Verification items for the finished model (mm, model axes). A direction names the side the tool comes from. Round coordinates to 2 decimals unless told otherwise and drop trailing zeros. Order: outer loops, then holes, each group sorted by start corner. A loop starts at its lowest first (then second) coordinate and runs counter-clockwise, first axis right, second up. Notation, with made-up numbers: (81.5, 10.5) -> (85.5, 10.5) arc R14 ccw to (85.5, 15.5) -> close; hole circle Ø9 at (1.25, -24). An arc over 180 degrees is marked (long way). Put each result on its own line as item: value.
```python
from build123d import *

# Parameters (mm, degrees)
SKETCH1_R           = 2.4765
BOSS_EXTRUDE1_DEPTH = 9.525
SKETCH2_R           = 3.9624
BOSS_EXTRUDE2_DEPTH = 2.38125
CUT_EXTRUDE1_DEPTH  = 2.286
FILLET1_R           = 1.5875


with BuildPart() as part:
    # Sketch1 → Boss-Extrude1 (new body)
    with BuildSketch(Plane(origin=(0, 0, 0), x_dir=(1, 0, 0), z_dir=(0, 1, 0))):
        with Locations(Location((0, 0, 0), (0, 0, 90))):
            Circle(SKETCH1_R)
    extrude(amount=BOSS_EXTRUDE1_DEPTH)

    # Sketch2 → Boss-Extrude2 (add)
    with BuildSketch(Plane.XZ):
        with Locations(Location((0, 0, 0), (0, 0, 90))):
            Circle(SKETCH2_R)
    extrude(amount=BOSS_EXTRUDE2_DEPTH)

    # Sketch3 → Cut-Extrude1 (cut)
    with BuildSketch(Plane.XZ.offset(2.38125)):
        Polygon((2.062222993, 0), (1.031111496, 1.7859375), (-1.031111496, 1.7859375), (-2.062222993, 0), (-1.031111496, -1.7859375), (1.031111496, -1.7859375), align=None)
    extrude(amount=-CUT_EXTRUDE1_DEPTH, mode=Mode.SUBTRACT)

    # Fillet1
    fillet1_edges = [part.edges().sort_by_distance(p)[0] for p in [
        (0, -2.38125, -3.9624),
    ]]
    fillet(fillet1_edges, radius=FILLET1_R)


solid = part.part
```
Item 1: Depth check by flat-ended pin: pin 1 Ø1.5 at (y, z) = (3, 2.5) entering from -X; pin 2 Ø3 at (y, z) = (3.5, 0.5) entering from -X; pin 3 Ø2.5 at (x, y) = (-0.5, -1.5) entering from -Z; pin 4 Ø1 at (x, y) = (1, 4) entering from +Z. Enter the tip coordinate at first touch or a pass-through.
Geometry check:
pin 1: x = -1.75
pin 2: x = -2.48
pin 3: z = -3.96
pin 4: z = 2.43
Item 2: Sectioned sample at B-B, the plane y = 4.5. Record the boundary of the cut face in (x, z), then the cut area to 3 significant figures.
Geometry check:
outline: circle Ø4.95 at (0, 0)
area: 19.3 mm2
Item 3: Sectioned sample at A-A, the plane x = 0. Record the boundary of the cut face in (y, z) (1 decimal), then the cut area to 3 significant figures.
Geometry check:
outline: (-2.4, -2.4) arc R1.6 ccw to (-0.8, -4) -> (0, -4) -> (0, -2.5) -> (9.5, -2.5) -> (9.5, 2.5) -> (0, 2.5) -> (0, 4) -> (-0.8, 4) arc R1.6 ccw to (-2.4, 2.4) -> (-2.4, 1.8) -> (-0.1, 1.8) -> (-0.1, -1.8) -> (-2.4, -1.8) -> close
area: 56.8 mm2
Item 4: Tool access check on faces 4 (the face through (-0.744, 4.696, -2.362)), 5 (the face through (1.75, -2.381, 0.87)), 6 (the face through (-1.554, -1.254, -0.88)). Record the directions out of +Z, -Z, +X, -X, +Y, -Y that give a thin tool (end or side, any length) a straight path to the whole face; none if there is none.
Geometry check:
face 4: +Y
face 5: +Z, -Z, +X, -X, -Y
face 6: -Y
Item 5: Material ranges on line 1 along X through (y, z) = (-0.75, -1); line 2 along Y through (x, z) = (-1.75, 0) (3 decimals); line 3 along Z through (x, y) = (0.25, -0.25), recorded low to high.
Geometry check:
line 1: -3.83 to -1.48, 1.48 to 3.83
line 2: -0.095 to 9.525
line 3: -3.95 to -1.79, 1.79 to 3.95
Item 6: Release check for a two-part mould opening along X. For faces 1 (the face through (-2, 0, 2)), 2 (the face through (1.539, -1.254, -0.905)), 3 (the face through (-3.93, -0.39, -0.52)) record: pulls with the +X half, pulls with the -X half, needs draft (parallel to the pull), parting line crosses it, or undercut.
Geometry check:
face 1: needs draft
face 2: undercut
face 3: parting line crosses it
